The drawing under review shows one solid part. Ordinate dimensions are in mm from its lowest x, y, z. Round coordinates to 2 decimals unless told otherwise and drop trailing zeros. Loops run counter-clockwise (first coordinate to the right, second up) from the corner with the lowest first, then second, coordinate; pieces in that order, holes last. Notation, with made-up numbers: M 1.5,-15 L 50.5,-15 A18 cw 50.5,4 Z; hole C 37,-13.75 d8. An arc over 180 degrees is marked long. Use a Markdown table: item, result.
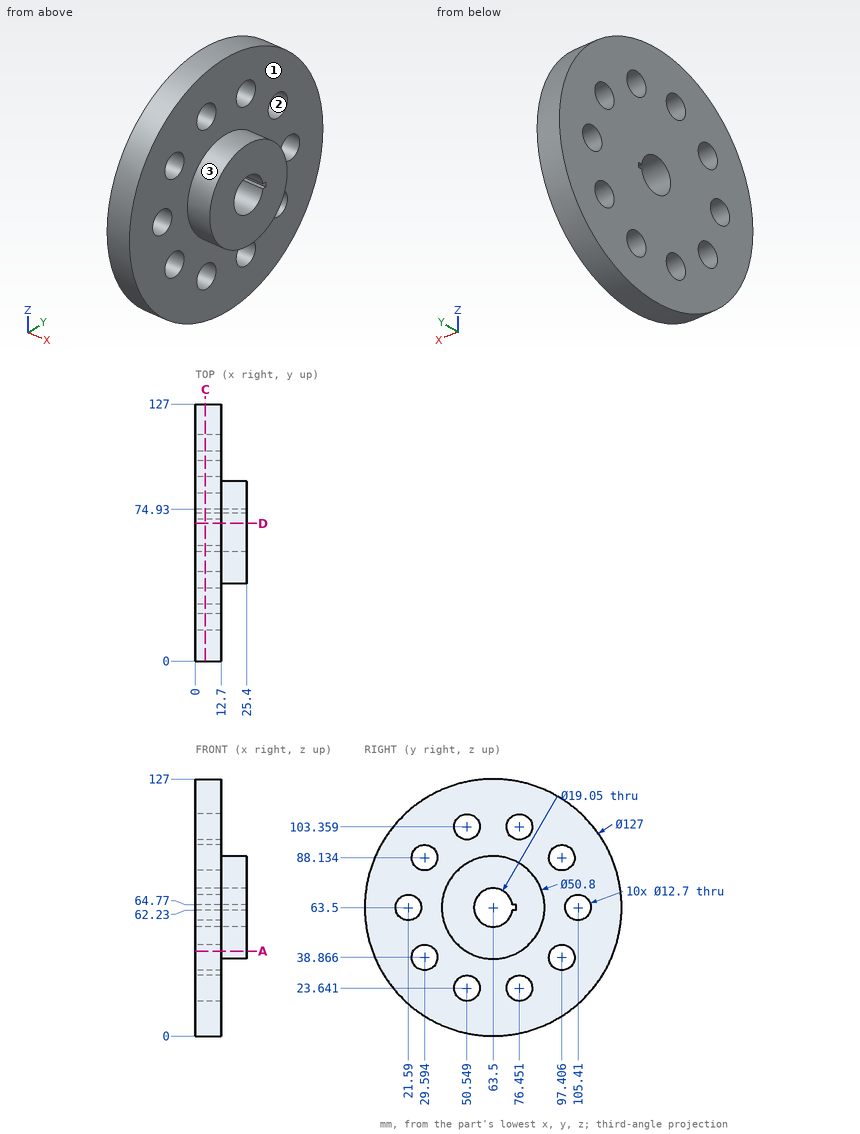
1. Wall thickness on line 1 along Y through (x, z) = (6.5, 84.5); line 2 along Y through (x, z) = (8.5, 33) (1 decimal); line 3 along Z through (x, y) = (1.25, 78): over which ranges is each line inside the solid? List them lowest first. Write a range as from..to.
Check values:
| item | result |
|---|---|
| line 1 | y = 3.57..24.39, 34.8..92.2, 102.61..123.43 |
| line 2 | y = 7.8..27.2, 32..95, 99.8..119.2 |
| line 3 | z = 1.68..17.48, 29.8..97.2, 109.52..125.32 |
2. Insertion check: pin 1 (4 mm diameter, centred on x = 19, y = 41, fed in from -Z); pin 2 (1.6 mm diameter, centred on x = 19, y = 73.5, fed in from +Z) (1 decimal); pin 3 (14.5 mm diameter, centred on y = 29.59, z = 88.13, fed in from +X). Each pin has a flat end and moves straight along its axis. Give the tip position at first contact, or say it passes through.
Check values:
| item | result |
|---|---|
| pin 1 | stops at z = 48.5 |
| pin 2 | stops at z = 87.2 |
| pin 3 | stops at x = 12.7 |
3. Take a section at C-C on x = 5. Count the separate pieces of the cut face and the enclosed holes in it, and give its area (3 significant figures).
Check values:
| item | result |
|---|---|
| separate pieces | 1 |
| enclosed holes | 11 |
| area | 11,100 mm² |
4. Take a section at A-A on z = 42. Give the boundary of the cut face in (x, y), and give its area (3 significant figures).
Check values:
| item | result |
|---|---|
| outline | M 0,3.75 L 12.7,3.75 L 12.7,24.07 L 0,24.07 Z; M 0,35.12 L 12.7,35.12 L 12.7,49.98 L 25.4,49.98 L 25.4,77.02 L 12.7,77.02 L 12.7,91.88 L 0,91.88 Z; M 0,102.93 L 12.7,102.93 L 12.7,123.25 L 0,123.25 Z |
| area | 1,580 mm² |
5. Take a section at D-D on y = 68. Give the boundary of the cut face in (x, z) (1 decimal).
Check values:
| item | result |
|---|---|
| outline | M 0,0.2 L 12.7,0.2 L 12.7,38.5 L 25.4,38.5 L 25.4,55.1 L 0,55.1 Z; M 0,71.9 L 25.4,71.9 L 25.4,88.5 L 12.7,88.5 L 12.7,126.8 L 0,126.8 Z |
6. The part is to be moulded in two halves that separate along Z. For the marked faces 1, 2 and 3, say which applies: pulls with the +Z half, pulls with the -Z half, needs draft (parallel to the pull), parting line crosses it, or undercut.
Check values:
| item | result |
|---|---|
| face 1 | needs draft |
| face 2 | undercut |
| face 3 | parting line crosses it |
